Study the drawing (mm; zero at the part's minimum x, y, z) and answer. A direction names the side the tool comes from. Coordinates: 2 decimals unless noted, no trailing zeros. Order: outer loops, then holes, each group sorted by start corner. A loop starts at its lowest first (then second) coordinate and runs counter-clockwise, first axis right, second up. Notation, with made-up numbers: (-25.5, 68) -> (15.5, 68) arc R17 ccw to (15.5, 72) -> close; hole circle Ø4 at (27.5, 70). An arc over 180 degrees is marked (long way). Write each question's results on one line, items separated by ' | '. Start each with the question number.
(1) The part is cut by section A-A, the plane y = 51.6. Give the vertices of the cut face in (x, z), then the cut area to 3 significant figures.
(2) Determine the mould class of the marked faces 1, 2, 3 and 4 for opening direction Y: +Y half, -Y half, draft (parallel to the pull), parting line (faces both ways), or undercut.
(3) Straight lines are drawn through the part: L1, parallel to X at y = 51.5, z = 4.5; L2, parallel to Y at x = 59.6, z = 12; L3, parallel to Y at x = 65, z = 6.75. For each, find the intervals that lie inside material, in ascending order.
(4) A tool of negligible diameter and unlimited length cuts with its end or side. For the marked faces 5, 6, 7, 8 and 9, from which of +Z, -Z, +X, -X, +Y, -Y can it reach the whole face along a straight path? Write none if from no direction.
(5) Given pin 1 (2.5 mm diameter, centred on x = 2.5, z = 10.5, fed in from -Y); pin 2 (12 mm diameter, centred on y = 41.5, z = 13, fed in from -X); pin 3 (3.5 mm diameter, centred on y = 3.5, z = 13.5, fed in from +X), each flat-ended and moving along its own axis, determine where each tip first touches the part or whether it passes through.
(6) The part is cut by section D-D, the plane y = 20. Give the vertices of the cut face in (x, z).
(7) The part is cut by section C-C, the plane z = 11.75. Give the vertices of the cut face in (x, y), then the cut area to 3 significant figures.
(8) The part is cut by section B-B, the plane x = 64.5. Give the vertices of the cut face in (y, z).
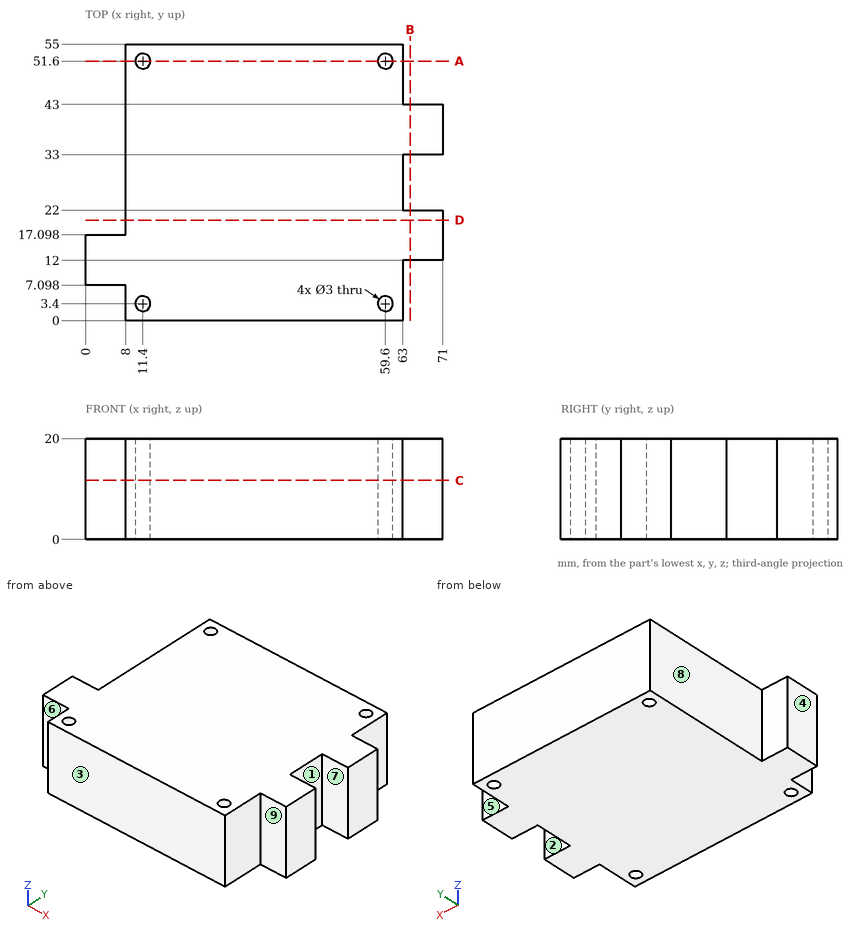
Established:
1) outline: (8, 0) -> (9.9, 0) -> (9.9, 20) -> (8, 20) -> close; (12.9, 0) -> (58.1, 0) -> (58.1, 20) -> (12.9, 20) -> close; (61.1, 0) -> (63, 0) -> (63, 20) -> (61.1, 20) -> close | area: 980 mm^2
2) face 1: undercut | face 2: undercut | face 3: -Y half | face 4: draft
3) L1: x = 8 to 9.9, 12.9 to 58.1, 61.1 to 63 | L2: y = 0 to 1.9, 4.9 to 50.1, 53.1 to 55 | L3: y = 12 to 22, 33 to 43
4) face 5: +Z, -Z, +X, +Y | face 6: +Z, -Z, -X, -Y | face 7: +Z, -Z, +X | face 8: +Z, -Z, -X, +Y | face 9: +Z, -Z, +X, -Y
5) pin 1: stops at y = 7.1 | pin 2: stops at x = 8 | pin 3: stops at x = 63
6) outline: (8, 0) -> (71, 0) -> (71, 20) -> (8, 20) -> close
7) outline: (0, 7.1) -> (8, 7.1) -> (8, 0) -> (63, 0) -> (63, 12) -> (71, 12) -> (71, 22) -> (63, 22) -> (63, 33) -> (71, 33) -> (71, 43) -> (63, 43) -> (63, 55) -> (8, 55) -> (8, 17.1) -> (0, 17.1) -> close; hole circle Ø3 at (11.4, 3.4); hole circle Ø3 at (11.4, 51.6); hole circle Ø3 at (59.6, 3.4); hole circle Ø3 at (59.6, 51.6) | area: 3,240 mm^2
8) outline: (12, 0) -> (22, 0) -> (22, 20) -> (12, 20) -> close; (33, 0) -> (43, 0) -> (43, 20) -> (33, 20) -> close
